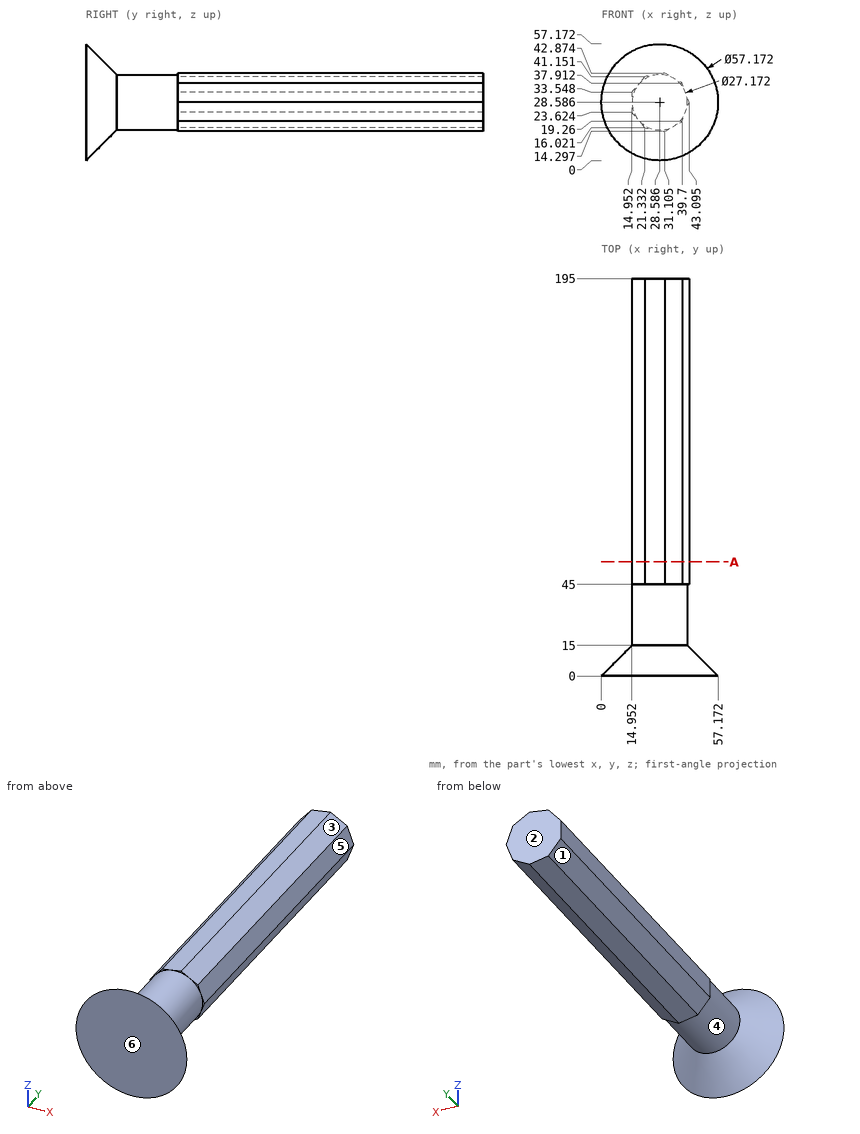
Study the drawing (mm; zero at the part's minimum x, y, z) and answer. A direction names the side the tool comes from. Coordinates: 2 decimals unless noted, no trailing zeros. Loops run counter-clockwise (first coordinate to the right, second up) from the corner with the lowest first, then second, coordinate; pieces in that order, holes last. Notation, with made-up numbers: M -11,79.25 L 18,79.25 A19 cw 18,91.25 Z; hole C -22,24 d3. An arc over 180 degrees is marked long. Answer in a Markdown table with one row per item.
1) Determine the mould class of the marked faces 4, 5 and 6 for opening direction Y: released by +Y, released by -Y, zero draft, split by the parting line, or undercut.
Answers below:
| item | result |
|---|---|
| face 4 | undercut |
| face 5 | zero draft |
| face 6 | released by -Y |
2) Find the intervals of material crossed by probe 1 along Z at (x, y) = (27, 112); probe 2 along Z at (x, y) = (37, 138.5); probe 3 along X at (y, z) = (142.5, 34) (1 decimal), in increasing order.
Answers below:
| item | result |
|---|---|
| probe 1 | 15.02 to 42.15 |
| probe 2 | 17.7 to 39.47 |
| probe 3 | 15.3 to 41.1 |
3) Find section A-A (y = 56). Determine the outline of the cut face in (x, z) (1 decimal).
Answers below:
| item | result |
|---|---|
| outline | M 15,23.6 L 21.3,16 L 31.1,14.3 L 39.7,19.3 L 43.1,28.6 L 39.7,37.9 L 31.1,42.9 L 21.3,41.2 L 15,33.5 Z |
4) Which of the six approach directions +Z, -Z, +X, -X, +Y, -Y give full straight-line access (tool end or side, diameter ignored) to the marked faces 1, 2 and 3?
Answers below:
| item | result |
|---|---|
| face 1 | -Z, -X, +Y |
| face 2 | +Z, -Z, +X, -X, +Y |
| face 3 | +Z, +X, +Y |
5) Given pin 1 (4 mm diameter, centred on x = 38, y = 72, fed in from +Z); pin 2 (3 mm diameter, centred on x = 36.5, y = 159, fed in from -Z) (1 decimal); pin 3 (11 mm diameter, centred on y = 95, z = 26.5, fed in from -X), each flat-ended and moving along its own axis, determine where each tip first touches the part or whether it passes through.
Answers below:
| item | result |
|---|---|
| pin 1 | z = 40.05 |
| pin 2 | z = 16.5 |
| pin 3 | x = 14.95 |
